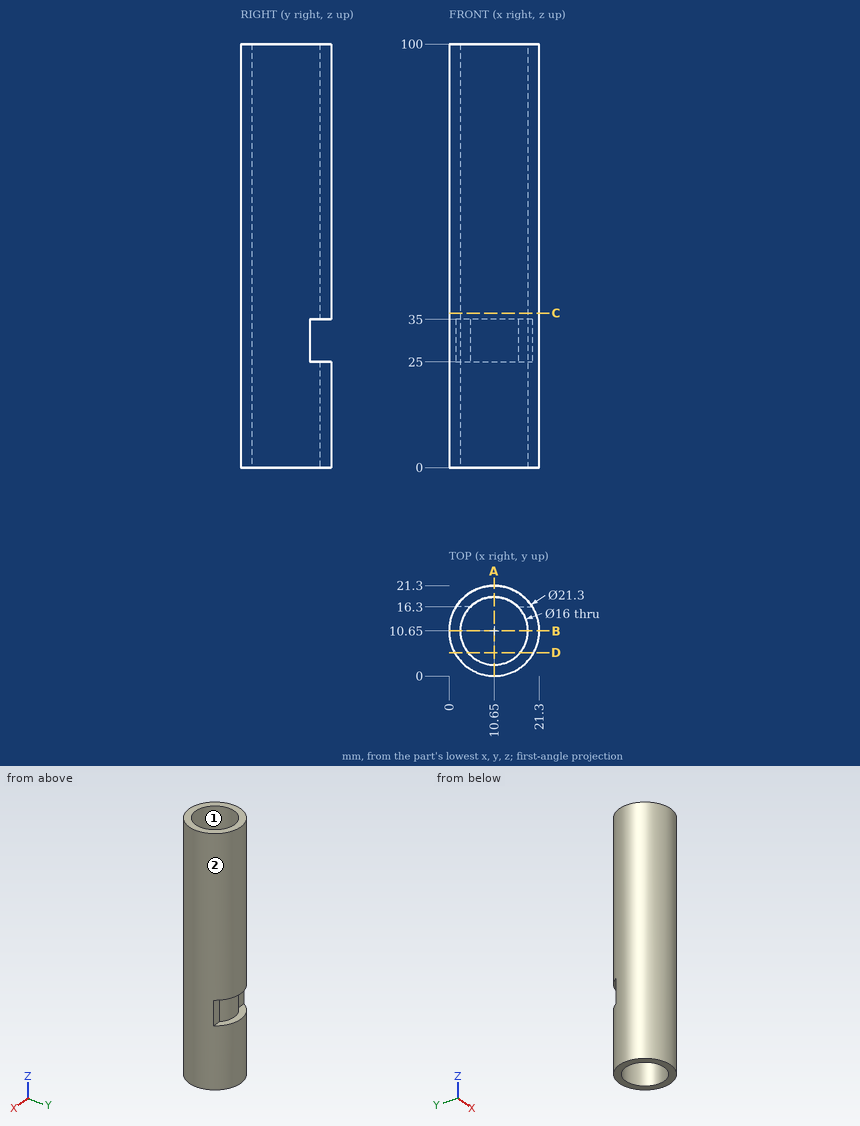
Can you work these out from the drawing? Everything is in mm from the part's minimum corner. Round coordinates to 2 decimals unless told otherwise and drop trailing zeros. Order: outer loops, then holes, each group sorted by start corner. A loop starts at its lowest first (then second) coordinate and runs counter-clockwise, first axis right, second up. Notation, with made-up numbers: M 6,80 L 49,80 A16 cw 49,98 Z; hole C 3,66 d4. An arc over 180 degrees is marked long. Answer as CSV lines item,"result".
Item 1: Imagine slicing it at A-A on x = 10.65. List the corners of the cut face in (y, z) for me.
From the geometry:
outline,"M 0,0 L 2.65,0 L 2.65,100 L 0,100 Z; M 18.65,0 L 21.3,0 L 21.3,25 L 18.65,25 Z; M 18.65,35 L 21.3,35 L 21.3,100 L 18.65,100 Z"
Item 2: For pin 1 (10 mm diameter, centred on y = 3, z = 65, fed in from -X); pin 2 (4 mm diameter, centred on x = 16, z = 14.5, fed in from +Y); pin 3 (3 mm diameter, centred on y = 15, z = 38.5, fed in from -X), each with a flat end and sliding along its axis, tell me the tip position at first contact or that it passes through.
From the geometry:
pin 1,"x = 0.33"
pin 2,"y = 20.76"
pin 3,"x = 0.39"
Item 3: Imagine slicing it at C-C on z = 36.5. List the corners of the cut face in (x, y) for me.
From the geometry:
outline,"C 10.65,10.65 d21.3; hole C 10.65,10.65 d16"
Item 4: We'd pull the mould along Y, two halves only. Please class the marked faces 1 and 2: +Y half, -Y half, draft (parallel to the pull), parting line (faces both ways), or undercut.
From the geometry:
face 1,"undercut"
face 2,"parting line"
Item 5: Imagine slicing it at B-B on y = 10.65. List the corners of the cut face in (x, z) for me, and give its area (3 significant figures).
From the geometry:
outline,"M 0,0 L 2.65,0 L 2.65,100 L 0,100 Z; M 18.65,0 L 21.3,0 L 21.3,100 L 18.65,100 Z"
area,"530 mm2"
Item 6: Imagine slicing it at D-D on y = 5.5. List the corners of the cut face in (x, z) for me, and give its area (3 significant figures).
From the geometry:
outline,"M 1.33,0 L 4.53,0 L 4.53,100 L 1.33,100 Z; M 16.77,0 L 19.97,0 L 19.97,100 L 16.77,100 Z"
area,"640 mm2"
Item 7: Please list where these lines run through material, in increasing order: L1, parallel to Y at x = 10.65, z = 55; L2, parallel to Y at x = 10.65, z = 29. Write a range as [from, to].
From the geometry:
L1,"[0, 2.65], [18.65, 21.3]"
L2,"[0, 2.65]"
